from build123d import *

# Parameters (mm, degrees)
F0_R     = 34
F0_R_2   = 20
F1_DEPTH = 15
F2_SIZE  = 2
F5_D     = 6.6
F5_DEPTH = 15
F5_START = 0.1605261
F5_TIP   = 1.9828400428


with BuildPart() as f1:
    # F0 (on Front) → F1 (new body)
    with BuildSketch(Plane.XZ):
        Circle(F0_R)
        Circle(F0_R_2, mode=Mode.SUBTRACT)
    extrude(amount=F1_DEPTH)

    # F2
    f2_edges = [f1.edges().sort_by_distance(p)[0] for p in [
        (-34, 0, 0),
        (-34, -15, 0),
    ]]
    chamfer(f2_edges, length=F2_SIZE)

    # F5
    # its depths count from where the whole tool has entered the part; down to there all is cleared
    with Locations(Plane.YZ.offset(34).offset(-F5_START)):
        with Locations((-7.5, 0)):
            Hole(F5_D / 2, depth=F5_DEPTH)
            with Locations((0, 0, -(F5_DEPTH + F5_TIP / 2))):  # 118° drill point
                Cone(0, F5_D / 2, F5_TIP, mode=Mode.SUBTRACT)


solid = f1.part
Can you work these out from the model? Positions are in its coordinate system, mm. Coordinates: 2 decimals unless noted, no trailing zeros. Write each loop counter-clockwise with the first axis right and the second up, starting at its lowest first coordinate (ties: lowest second). Pieces come first, ordered by that corner, then holes. Notation, with made-up numbers: (-16.5, -38) -> (-11.5, -38) arc R31 cw to (-11.5, -3) -> close; hole circle Ø11 at (-2.75, 65.25). An arc over 180 degrees is marked (long way). Answer as CSV lines item,"result".
1) If we section it at C-C on y = -5.25: Please give me the cut outline in (x, z).
Check result:
outline,"(19.85, -2.41) arc R20 cw (long way) to (19.85, 2.41) -> (33.91, 2.41) arc R34 ccw (long way) to (33.91, -2.41) -> close"
2) If we section it at A-A on x = 0: Please give me the cut outline in (y, z).
Check result:
outline,"(-15, -32) -> (-13, -34) -> (-2, -34) -> (0, -32) -> (0, -20) -> (-15, -20) -> close; (-15, 20) -> (0, 20) -> (0, 32) -> (-2, 34) -> (-13, 34) -> (-15, 32) -> close"
3) Will these pins go through, and if not, where does the flat tip stop? P1, Ø4, axis at x = 26.5, y = -10.5, coming from the +Z side; P2, Ø4, axis at y = -8.5, z = 13.5, coming from the -X side; P3, Ø2, axis at y = -10.5, z = 25.5, coming from the -X side; P4, Ø6, axis at x = -14, z = 2, coming from the +Y side.
Check result:
P1,"z = 23.57"
P2,"x = -32"
P3,"x = -23.57"
P4,"through"
4) If we mould it in two halves opening along Y, with no side actions, what happens to faces 1 (the flat face through (14, -15, 15)), 2 (the cylindrical face through (26.763, -4.881, -2.008)), 3 (the flat face through (14, 0, 15))? For each: +Y half, -Y half, draft (parallel to the pull), parting line (faces both ways), or undercut.
Check result:
face 1,"-Y half"
face 2,"undercut"
face 3,"+Y half"
5) If I drill on line 1 (Y direction, x = 24, z = 0); line 2 (Y direction, x = 28, z = 1); line 3 (X direction, y = -9.25, z = -11), over which ranges is the centre line in solid material (lowest first)? Write a range as from..to.
Check result:
line 1,"-15..-10.8, -4.2..0"
line 2,"-15..-10.64, -4.36..0"
line 3,"-32.17..-16.7, 16.7..32.17"
6) If we section it at B-B on z = 0: Please give me the cut outline in (x, y).
Check result:
outline,"(-34, -13) -> (-32, -15) -> (-20, -15) -> (-20, 0) -> (-32, 0) -> (-34, -2) -> close; (20, -15) -> (32, -15) -> (34, -13) -> (34, -10.8) -> (20, -10.8) -> close; (20, -4.2) -> (34, -4.2) -> (34, -2) -> (32, 0) -> (20, 0) -> close"
